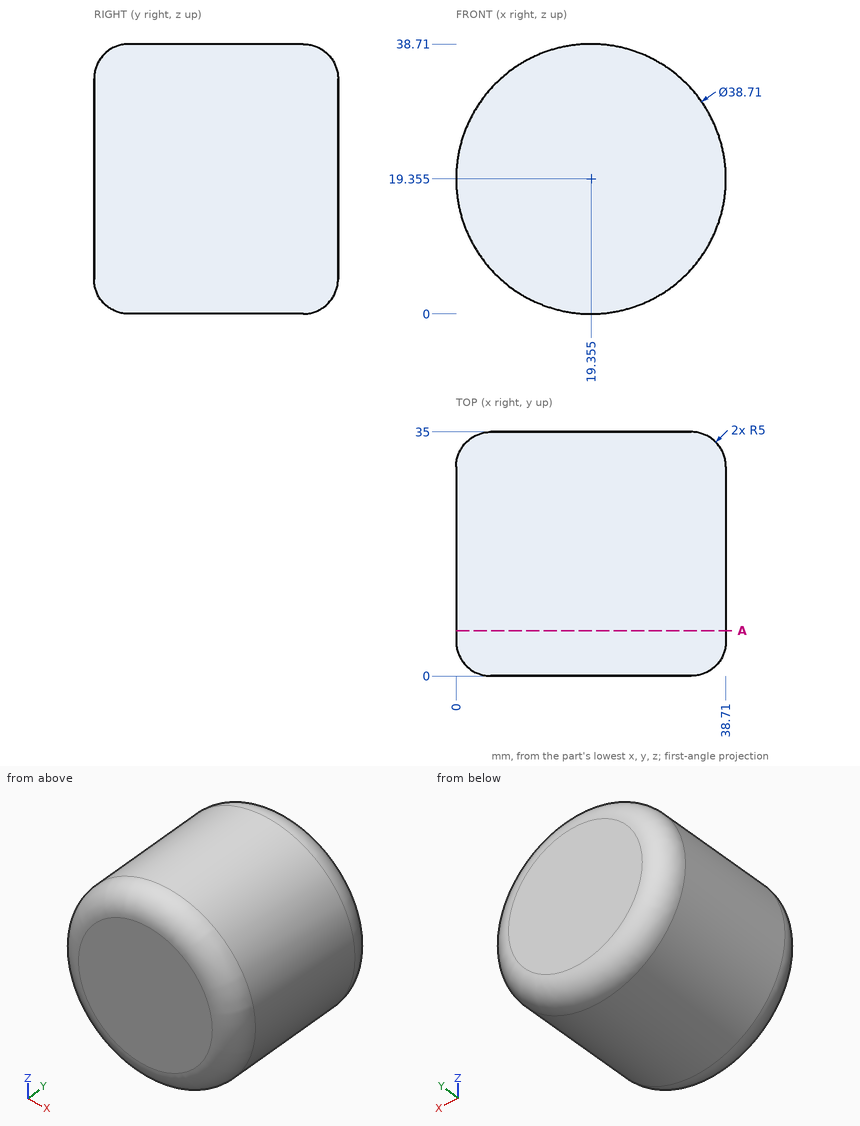
Could you check a few things on this drawing? It's one solid part, dimensions in mm from its lowest x, y, z. Give positions to 0.01 mm unless a question says otherwise; leave off trailing zeros. Order: outer loops, then holes, each group sorted by start corner. A loop starts at its lowest first (then second) coordinate and runs counter-clockwise, first axis right, second up. Notation, with made-up numbers: (-39.5, 10) - (-5.5, 10) arc R26 cw to (-5.5, 35) - close; hole circle Ø4 at (61, 16.25). An arc over 180 degrees is marked (long way). Answer as a JSON object with one key per item and string values. Group by question number.
Item 1: If we section it at A-A on y = 6.5: Please give me the cut outline in (x, z) (1 decimal).
Item 2: For P1, Ø1, axis at x = 30, y = 25.5, coming from the +Z side; P2, Ø2, axis at y = 20.5, z = 7, coming from the +X side; P3, Ø10, axis at x = 12.5, y = 31, coming from the -Z side, each with a flat end and sliding along its axis, tell me the tip position at first contact or that it passes through.
Item 3: Please list where these lines run through material, in increasing order: probe 1 along Y at (x, z) = (32, 12); probe 2 along Z at (x, y) = (19.5, 16.5); probe 3 along X at (y, z) = (11, 23).
Result set:
{
 "1": {"outline": "circle Ø38.7 at (19.4, 19.4)"},
 "2": {"P1": "z = 35.84", "P2": "x = 35.03", "P3": "z = 0.1"},
 "3": {"probe 1": "0.01 to 34.99", "probe 2": "0 to 38.71", "probe 3": "0.35 to 38.36"}
}
